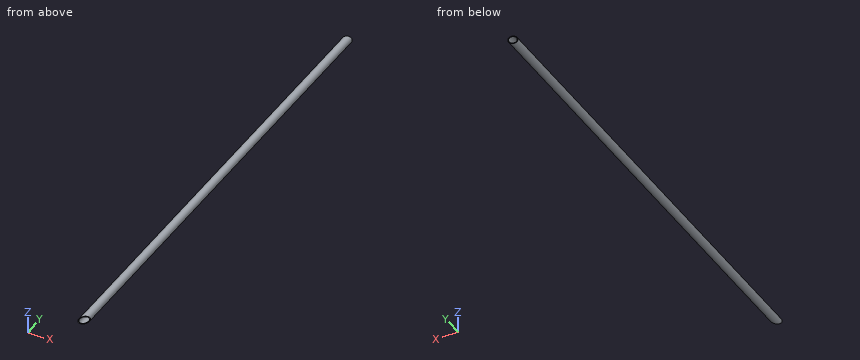
from build123d import *

# Parameters (mm, degrees)
F0_R          = 21.2
F0_R_2        = 17.95
F1_DEPTH      = 2500
F3_DEPTH      = 21.201
F3_DEPTH_BACK = 21.201
F5_DEPTH      = 21.201
F5_DEPTH_BACK = 21.201


with BuildPart() as f1:
    # F0 (on Front) → F1 (new body)
    with BuildSketch(Plane.XZ):
        Circle(F0_R)
        Circle(F0_R_2, mode=Mode.SUBTRACT)
    extrude(amount=F1_DEPTH)

    # F2 (on Top) → F3 (cut, two sides)
    with BuildSketch(Plane.XY) as f3_sk:
        Polygon((-21.2, 0), (-21.2, -16.8792704184), (21.2, 0), align=None)
    extrude(amount=-F3_DEPTH, mode=Mode.SUBTRACT)
    extrude(f3_sk.sketch, amount=F3_DEPTH_BACK, mode=Mode.SUBTRACT)

    # F4 (on Top) → F5 (cut, two sides)
    with BuildSketch(Plane.XY) as f5_sk:
        Polygon((21.2, -2500), (21.2, -2370.596422726), (-21.2, -2410.7125909795), (-21.2, -2500), align=None)
    extrude(amount=-F5_DEPTH, mode=Mode.SUBTRACT)
    extrude(f5_sk.sketch, amount=F5_DEPTH_BACK, mode=Mode.SUBTRACT)


solid = f1.part
Here's how the part is built. I have some questions about the finished solid (model axes, mm). Coordinates: 2 decimals unless noted, no trailing zeros. Order: outer loops, then holes, each group sorted by start corner. A loop starts at its lowest first (then second) coordinate and runs counter-clockwise, first axis right, second up. Notation, with made-up numbers: (14.25, -24.5) - (63.25, -24.5) arc R18 ccw to (63.25, -7.5) - close; hole circle Ø11 at (-15, 42). An arc over 180 degrees is marked (long way). Use CSV: the item, a comma, the result in double quotes. Start each with the question number.
1. Suppose I cut it at C-C on y = -444. List the corners of the cut face in (x, z) for me.
2. Please list where these lines run through material, in increasing order: line 1 (X direction, y = -513.5, z = 0); line 2 (Z direction, x = -4, y = -1035.5). Write a range as from..to.
3. Suppose I cut it at A-A on z = 0. List the corners of the cut face in (x, y) for me, then the cut area to 3 significant figures.
4. I'm going to push flat-ended pins straight in: pin 1 (5 mm diameter, centred on y = -1078.5, z = -12, fed in from +X); pin 2 (1.5 mm diameter, centred on y = -1314.5, z = -15, fed in from +X); pin 3 (8 mm diameter, centred on x = 16, y = -1949.5, fed in from -Z). Where does each tip first touch, or does it pass through?
5. Suppose I cut it at B-B on x = 1.5. List the corners of the cut face in (y, z) for me, then the cut area to 3 significant figures.
Output:
1,outline,"circle Ø42.4 at (0, 0); hole circle Ø35.9 at (0, 0)"
2,line 1,"x = -21.2..-17.95, 17.95..21.2"
2,line 2,"z = -20.82..-17.5, 17.5..20.82"
3,outline,"(-21.2, -2410.71) - (-17.95, -2407.64) - (-17.95, -15.59) - (-21.2, -16.88) - close; (17.95, -2373.67) - (21.2, -2370.6) - (21.2, 0) - (17.95, -1.29) - close"
3,area,"15,500 mm2"
4,pin 1,"stops at x = 18.95"
4,pin 2,"stops at x = 15.7"
4,pin 3,"stops at z = -17.48"
5,outline,"(-2389.24, -21.15) - (-7.84, -21.15) - (-7.84, -17.89) - (-2389.24, -17.89) - close; (-2389.24, 17.89) - (-7.84, 17.89) - (-7.84, 21.15) - (-2389.24, 21.15) - close"
5,area,"15,500 mm2"
